Can you work these out from the model? Positions are in its coordinate system, mm. A direction names the side the tool comes from. Give positions to 0.01 mm unless a question says otherwise; leave off trailing zeros. Order: outer loops, then holes, each group sorted by start corner. A loop starts at its lowest first (then second) coordinate and runs counter-clockwise, first axis right, second up. Notation, with made-up numbers: (69.5, 38.25) - (90.5, 38.25) arc R16 cw to (90.5, 66.25) - close; hole circle Ø9 at (6.25, 53). An arc over 180 degrees is marked (long way). Answer as a JSON object with one key per item and string values.
```python
from build123d import *

# Parameters (mm, degrees)
F0_W     = 600
F0_H     = 800
F0_R     = 6.552392
F0_W_2   = 560
F0_H_2   = 760
F1_DEPTH = 35
F2_R     = 6.552392
F3_DEPTH = 400
F4_W     = 600
F4_H     = 800
F5_DEPTH = 25


with BuildPart() as f1:
    # F0 (on Top) → F1 (new body)
    with BuildSketch(Plane.XY):
        with Locations((-7, -51)):
            Rectangle(F0_W, F0_H)
        with Locations((-297, -433.404595)):
            Circle(F0_R, mode=Mode.SUBTRACT)
        with Locations((-297, -375.404595)):
            Circle(F0_R, mode=Mode.SUBTRACT)
        with Locations((-297, -317.404595)):
            Circle(F0_R, mode=Mode.SUBTRACT)
        with Locations((-297, -259.404595)):
            Circle(F0_R, mode=Mode.SUBTRACT)
        with Locations((-297, -201.404595)):
            Circle(F0_R, mode=Mode.SUBTRACT)
        with Locations((-297, -143.404595)):
            Circle(F0_R, mode=Mode.SUBTRACT)
        with Locations((-297, -85.404595)):
            Circle(F0_R, mode=Mode.SUBTRACT)
        with Locations((283, -433.404595)):
            Circle(F0_R, mode=Mode.SUBTRACT)
        with Locations((283, -375.404595)):
            Circle(F0_R, mode=Mode.SUBTRACT)
        with Locations((283, -317.404595)):
            Circle(F0_R, mode=Mode.SUBTRACT)
        with Locations((283, -259.404595)):
            Circle(F0_R, mode=Mode.SUBTRACT)
        with Locations((283, -201.404595)):
            Circle(F0_R, mode=Mode.SUBTRACT)
        with Locations((283, -143.404595)):
            Circle(F0_R, mode=Mode.SUBTRACT)
        with Locations((283, -85.404595)):
            Circle(F0_R, mode=Mode.SUBTRACT)
        with Locations((-297, -27.404595)):
            Circle(F0_R, mode=Mode.SUBTRACT)
        with Locations((-297, 30.595405)):
            Circle(F0_R, mode=Mode.SUBTRACT)
        with Locations((-297, 88.595405)):
            Circle(F0_R, mode=Mode.SUBTRACT)
        with Locations((-297, 146.595405)):
            Circle(F0_R, mode=Mode.SUBTRACT)
        with Locations((-297, 204.595405)):
            Circle(F0_R, mode=Mode.SUBTRACT)
        with Locations((-297, 262.595405)):
            Circle(F0_R, mode=Mode.SUBTRACT)
        with Locations((-297, 320.595405)):
            Circle(F0_R, mode=Mode.SUBTRACT)
        with Locations((-7, -51)):
            Rectangle(F0_W_2, F0_H_2, mode=Mode.SUBTRACT)
        with Locations((283, -27.404595)):
            Circle(F0_R, mode=Mode.SUBTRACT)
        with Locations((283, 30.595405)):
            Circle(F0_R, mode=Mode.SUBTRACT)
        with Locations((283, 88.595405)):
            Circle(F0_R, mode=Mode.SUBTRACT)
        with Locations((283, 146.595405)):
            Circle(F0_R, mode=Mode.SUBTRACT)
        with Locations((283, 204.595405)):
            Circle(F0_R, mode=Mode.SUBTRACT)
        with Locations((283, 262.595405)):
            Circle(F0_R, mode=Mode.SUBTRACT)
        with Locations((283, 320.595405)):
            Circle(F0_R, mode=Mode.SUBTRACT)
        with Locations((283, -433.404595)):
            Circle(F0_R)
        with Locations((283, -375.404595)):
            Circle(F0_R)
        with Locations((283, -317.404595)):
            Circle(F0_R)
        with Locations((283, -259.404595)):
            Circle(F0_R)
        with Locations((283, -201.404595)):
            Circle(F0_R)
        with Locations((283, -143.404595)):
            Circle(F0_R)
        with Locations((283, -85.404595)):
            Circle(F0_R)
        with Locations((283, -27.404595)):
            Circle(F0_R)
        with Locations((283, 30.595405)):
            Circle(F0_R)
        with Locations((283, 88.595405)):
            Circle(F0_R)
        with Locations((283, 146.595405)):
            Circle(F0_R)
        with Locations((283, 204.595405)):
            Circle(F0_R)
        with Locations((283, 262.595405)):
            Circle(F0_R)
        with Locations((283, 320.595405)):
            Circle(F0_R)
        with Locations((-297, 320.595405)):
            Circle(F0_R)
        with Locations((-297, 262.595405)):
            Circle(F0_R)
        with Locations((-297, 204.595405)):
            Circle(F0_R)
        with Locations((-297, 146.595405)):
            Circle(F0_R)
        with Locations((-297, 88.595405)):
            Circle(F0_R)
        with Locations((-297, 30.595405)):
            Circle(F0_R)
        with Locations((-297, -27.404595)):
            Circle(F0_R)
        with Locations((-297, -85.404595)):
            Circle(F0_R)
        with Locations((-297, -143.404595)):
            Circle(F0_R)
        with Locations((-297, -201.404595)):
            Circle(F0_R)
        with Locations((-297, -259.404595)):
            Circle(F0_R)
        with Locations((-297, -317.404595)):
            Circle(F0_R)
        with Locations((-297, -375.404595)):
            Circle(F0_R)
        with Locations((-297, -433.404595)):
            Circle(F0_R)
    extrude(amount=-F1_DEPTH)

    # F2 (on face) → F3 (join)
    with BuildSketch(Plane(origin=(0, 0, -35), x_dir=(1, 0, 0), z_dir=(0, 0, -1))):
        with Locations((-297, 433.404595)):
            Circle(F2_R)
        with Locations((-297, 143.404595)):
            Circle(F2_R)
        with Locations((-297, 375.404595)):
            Circle(F2_R)
        with Locations((-297, -204.595405)):
            Circle(F2_R)
        with BuildLine():
            ThreePointArc((-297, 33.956987), (-303.552392, 27.404595), (-297, 20.852203))
            Line((-297, 20.852203), (-297, 27.404595))
            Line((-297, 27.404595), (-297, 33.956987))
        make_face()
        with Locations((-297, -262.595405)):
            Circle(F2_R)
        with Locations((-297, -146.595405)):
            Circle(F2_R)
        with Locations((-297, 259.404595)):
            Circle(F2_R)
        with Locations((283, -88.595405)):
            Circle(F2_R)
        with BuildLine():
            ThreePointArc((-297, -24.043013), (-301.633241, -35.228646), (-290.447608, -30.595405))
            ThreePointArc((-290.447608, -30.595405), (-292.366759, -25.962164), (-297, -24.043013))
        make_face()
        with Locations((283, 85.404595)):
            Circle(F2_R)
        with Locations((283, -320.595405)):
            Circle(F2_R)
        with Locations((283, -204.595405)):
            Circle(F2_R)
        with Locations((283, -262.595405)):
            Circle(F2_R)
        with Locations((283, 143.404595)):
            Circle(F2_R)
        with Locations((283, 259.404595)):
            Circle(F2_R)
        with Locations((283, -146.595405)):
            Circle(F2_R)
        with Locations((283, 317.404595)):
            Circle(F2_R)
        with Locations((283, 201.404595)):
            Circle(F2_R)
        with Locations((283, -30.595405)):
            Circle(F2_R)
        with Locations((283, 27.404595)):
            Circle(F2_R)
        with BuildLine():
            ThreePointArc((-290.447608, 85.404595), (-301.633241, 90.037836), (-297, 78.852203))
            ThreePointArc((-297, 78.852203), (-292.366759, 80.771354), (-290.447608, 85.404595))
        make_face()
        with Locations((-297, 201.404595)):
            Circle(F2_R)
        with Locations((-297, -88.595405)):
            Circle(F2_R)
        with Locations((-297, 317.404595)):
            Circle(F2_R)
        with Locations((-297, -320.595405)):
            Circle(F2_R)
        with BuildLine():
            Line((-297, 27.404595), (-297, 20.852203))
            ThreePointArc((-297, 20.852203), (-292.366759, 22.771354), (-290.447608, 27.404595))
            ThreePointArc((-290.447608, 27.404595), (-292.366759, 32.037836), (-297, 33.956987))
            Line((-297, 33.956987), (-297, 27.404595))
        make_face()
        with Locations((283, 433.404595)):
            Circle(F2_R)
        with Locations((283, 375.404595)):
            Circle(F2_R)
    extrude(amount=F3_DEPTH)

    # F4 (on face) → F5 (join)
    with BuildSketch(Plane(origin=(0, 0, -435), x_dir=(1, 0, 0), z_dir=(0, 0, -1))):
        with Locations((-7, 51)):
            Rectangle(F4_W, F4_H)
    extrude(amount=F5_DEPTH)


solid = f1.part
```
Q1. I'm going to push a flat-ended pin straight in: pin 1 Ø8 at (y, z) = (-140, -373) entering from +X. Where does the tip first touch, or does it pass through?
Recorded:
{"pin 1": "stops at x = 289.55"}
Q2. If we section it at C-C, the plane y = -354: Please give me the cut outline in (x, z).
Recorded:
{"outline": "(-307, -460) - (293, -460) - (293, -435) - (-307, -435) - close; (-307, -35) - (-287, -35) - (-287, 0) - (-307, 0) - close; (273, -35) - (293, -35) - (293, 0) - (273, 0) - close"}
Q3. I need wall thicknesses on L1, parallel to X at y = -142.5, z = -379; L2, parallel to Y at x = -225, z = -20; L3, parallel to Z at x = -75, y = -194.5. Which ranges of each line are inside material? Lowest first, please.
Recorded:
{"L1": "x = -303.49 to -290.51, 276.51 to 289.49", "L2": "y = -451 to -431, 329 to 349", "L3": "z = -460 to -435"}
Q4. We'd pull the mould along Y, two halves only. Please class faces 1 (the face through (-307, -45, -447)), 2 (the face through (-11, -451, -447)), 3 (the face through (273, -56, -17)): released by +Y, released by -Y, zero draft, split by the parting line, or undercut.
Recorded:
{"face 1": "zero draft", "face 2": "released by -Y", "face 3": "undercut"}
Q5. If we section it at B-B, the plane z = -94.5: Count the separate pieces of the cut face and the enclosed holes in it, then the cut area to 3 significant figures.
Recorded:
{"separate pieces": "28", "enclosed holes": "0", "area": "3,780 mm^2"}
Q6. If we section it at A-A, the plane x = -66: Please give me the cut outline in (y, z).
Recorded:
{"outline": "(-451, -460) - (349, -460) - (349, -435) - (-451, -435) - close; (-451, -35) - (-431, -35) - (-431, 0) - (-451, 0) - close; (329, -35) - (349, -35) - (349, 0) - (329, 0) - close"}
Q7. Which directions (+Z, -Z, +X, -X, +Y, -Y) give clear straight access to the entire face, cutting with the end or side of a thin tool? Please do faces 4 (the face through (-287, -56, -17)), 5 (the face through (-297, -20, -35)), 6 (the face through (-307, -57, -17)).
Recorded:
{"face 4": "+Z", "face 5": "none", "face 6": "+Z, -Z, -X, +Y, -Y"}
